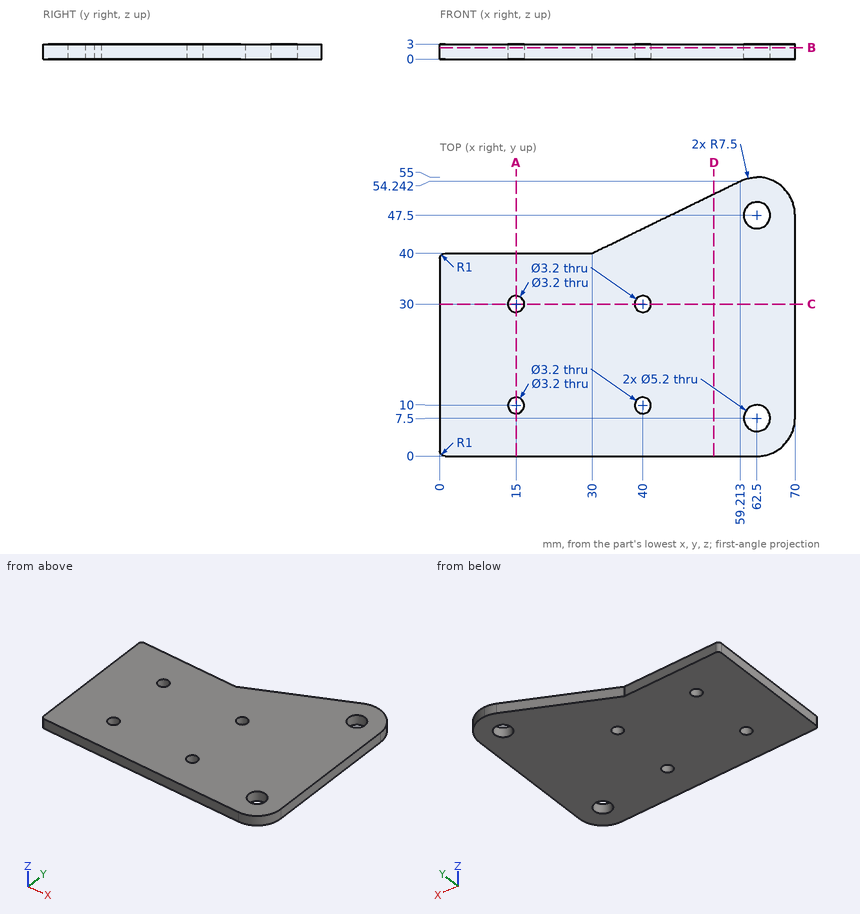
Check sheet for the drawn part. Datum: minimum x, y, z corner. Units: mm. Give positions to 0.01 mm unless a question says otherwise; leave off trailing zeros. Loops run counter-clockwise (first coordinate to the right, second up) from the corner with the lowest first, then second, coordinate; pieces in that order, holes last. Notation, with made-up numbers: (67, 8.25) - (123, 8.25) arc R19 ccw to (123, 12.25) - close; hole circle Ø2 at (27.5, 34.25). An arc over 180 degrees is marked (long way). Write each question's results on one line, items separated by ' | '.
1) Sectioned sample at A-A on x = 15. Record the boundary of the cut face in (y, z), plus the area to 3 significant figures.
Solution:
outline: (0, 0) - (8.4, 0) - (8.4, 3) - (0, 3) - close; (11.6, 0) - (28.4, 0) - (28.4, 3) - (11.6, 3) - close; (31.6, 0) - (40, 0) - (40, 3) - (31.6, 3) - close | area: 101 mm2
2) Sectioned sample at C-C on y = 30. Record the boundary of the cut face in (x, z), plus the area to 3 significant figures.
Solution:
outline: (0, 0) - (13.4, 0) - (13.4, 3) - (0, 3) - close; (16.6, 0) - (38.4, 0) - (38.4, 3) - (16.6, 3) - close; (41.6, 0) - (70, 0) - (70, 3) - (41.6, 3) - close | area: 191 mm2
3) Sectioned sample at D-D on x = 54. Record the boundary of the cut face in (y, z).
Solution:
outline: (0, 0) - (51.7, 0) - (51.7, 3) - (0, 3) - close
4) Sectioned sample at B-B on z = 2.3. Record the boundary of the cut face in (x, y).
Solution:
outline: (0, 1) arc R1 ccw to (1, 0) - (62.5, 0) arc R7.5 ccw to (70, 7.5) - (70, 47.5) arc R7.5 ccw to (59.21, 54.24) - (30, 40) - (1, 40) arc R1 ccw to (0, 39) - close; hole circle Ø3.2 at (15, 10); hole circle Ø3.2 at (15, 30); hole circle Ø3.2 at (40, 10); hole circle Ø3.2 at (40, 30); hole circle Ø5.2 at (62.5, 7.5); hole circle Ø5.2 at (62.5, 47.5)
5) Depth check by flat-ended pin: P1, Ø1.5, axis at x = 15.5, z = 2, coming from the +Y side. Enter the tip coordinate at first touch or a pass-through.
Solution:
P1: y = 40
6) Material ranges on L1, parallel to Y at x = 15, z = 0.7; L2, parallel to Y at x = 62.5, z = 2.35; L3, parallel to X at y = 7.5, z = 1.55, recorded low to high. Write a range as from..to.
Solution:
L1: 0..8.4, 11.6..28.4, 31.6..40 | L2: 0..4.9, 10.1..44.9, 50.1..55 | L3: 0..59.9, 65.1..70
